Answer from the drawing. Dimensions are ordinates in mm from the lowest x, y and z of the part. A direction names the side the tool comes from. Coordinates: 2 decimals unless noted, no trailing zeros. Write each loop counter-clockwise with the first axis right and the second up, starting at its lowest first coordinate (ties: lowest second). Pieces come first, ordered by that corner, then holes.
(1) Section A-A on y = 9.5 is taken. Write down the section's boundary in (x, z).
(2) Section D-D on x = 10 is taken. Write down the section's boundary in (y, z), then the cut area to 3 significant figures.
(3) Section B-B on x = 122 is taken. Write down the section's boundary in (y, z).
(4) Section C-C on z = 41.5 is taken. Write down the section's boundary in (x, y), then the cut area to 3 significant figures.
(5) The mould has two halves that part along X. Classify the marked faces 1, 2 and 3: +X half, -X half, draft (parallel to the pull), parting line (faces both ways), or undercut.
(6) Which of the six approach directions +Z, -Z, +X, -X, +Y, -Y give full straight-line access (tool end or side, diameter ignored) to the marked faces 4, 5 and 6?
(7) Given pin 1 (19 mm diameter, centred on x = 119.5, z = 56.5, fed in from -Y); pin 2 (3 mm diameter, centred on y = 2, z = 49, fed in from -X); pin 3 (3 mm diameter, centred on y = 2, z = 27, fed in from +X), each flat-ended and moving along its own axis, determine where each tip first touches the part or whether it passes through.
(8) Find the intervals of material crossed by probe 1 along X at (y, z) = (13.5, 70); probe 2 along Z at (x, y) = (12, 7.75); probe 3 along X at (y, z) = (19, 54), in increasing order.
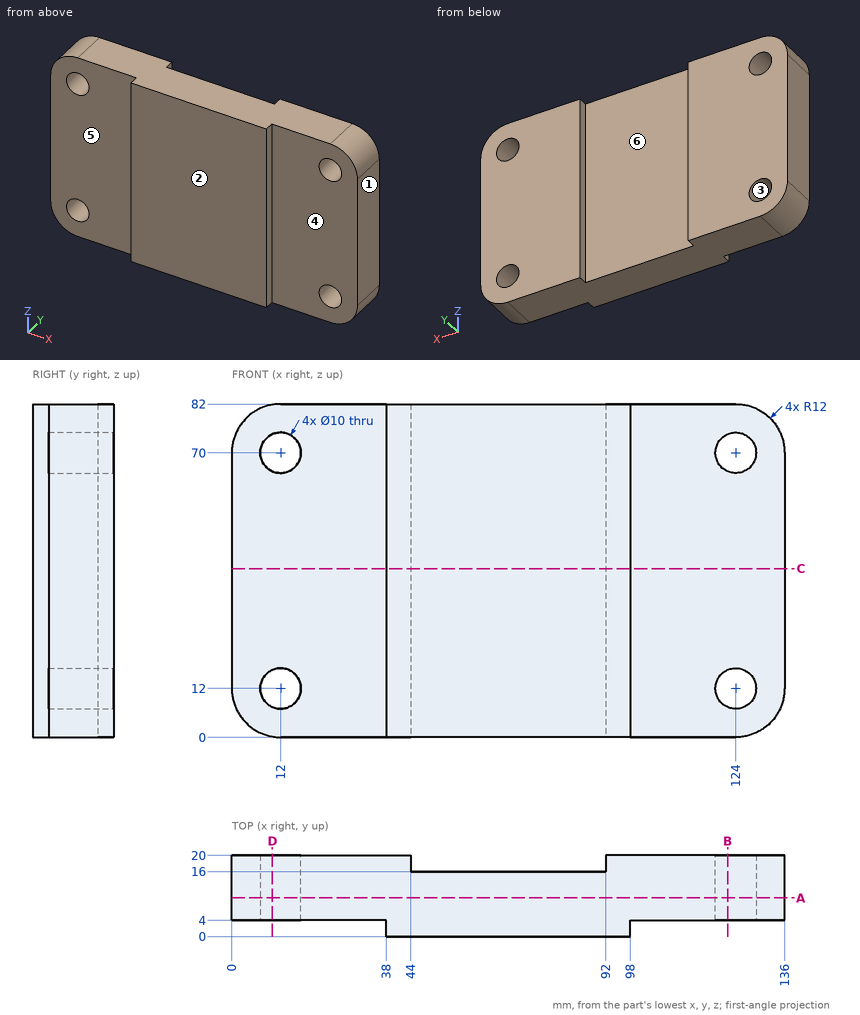
Response:
1. outline: (0, 12) arc R12 ccw to (12, 0) - (124, 0) arc R12 ccw to (136, 12) - (136, 70) arc R12 ccw to (124, 82) - (12, 82) arc R12 ccw to (0, 70) - close; hole circle Ø10 at (12, 12); hole circle Ø10 at (12, 70); hole circle Ø10 at (124, 12); hole circle Ø10 at (124, 70)
2. outline: (4, 0.17) - (20, 0.17) - (20, 7.42) - (4, 7.42) - close; (4, 16.58) - (20, 16.58) - (20, 65.42) - (4, 65.42) - close; (4, 74.58) - (20, 74.58) - (20, 81.83) - (4, 81.83) - close
2. area: 1,010 mm2
3. outline: (4, 0) - (20, 0) - (20, 7.42) - (4, 7.42) - close; (4, 16.58) - (20, 16.58) - (20, 65.42) - (4, 65.42) - close; (4, 74.58) - (20, 74.58) - (20, 82) - (4, 82) - close
4. outline: (0, 4) - (38, 4) - (38, 0) - (98, 0) - (98, 4) - (136, 4) - (136, 20) - (92, 20) - (92, 16) - (44, 16) - (44, 20) - (0, 20) - close
4. area: 2,220 mm2
5. face 1: +X half
5. face 2: draft
5. face 3: undercut
6. face 4: +Z, -Z, +X, -Y
6. face 5: +Z, -Z, -X, -Y
6. face 6: +Z, -Z, +Y
7. pin 1: stops at y = 4
7. pin 2: stops at x = 38
7. pin 3: stops at x = 98
8. probe 1: x = 0 to 7, 17 to 119, 129 to 136
8. probe 2: z = 0 to 7, 17 to 65, 75 to 82
8. probe 3: x = 0 to 44, 92 to 136
